The listing builds one solid part. Answer for the finished solid, in the listing's coordinates (mm). A direction names the side the tool comes from. Round coordinates to 2 decimals unless told otherwise and drop trailing zeros. Write each loop counter-clockwise with the first axis right and the second up, starting at its lowest first coordinate (ties: lowest second). Pieces come first, ordered by that corner, then holes.
Item 1: Find section A-A on x = 32. Give the vertices of the cut face in (y, z).
Item 2: Find section C-C on z = 63.5. Give the vertices of the cut face in (x, y).
Item 3: Find section B-B on z = -29.5. Give the vertices of the cut face in (x, y).
Item 4: Each of these flat-tipped pins is pushed along its axis until it touches: pin 1 (5 mm diameter, centred on x = -27, z = 65.5, fed in from -Y); pin 2 (1.1 mm diameter, centred on y = -1.5, z = 48.5, fed in from -X); pin 3 (1.5 mm diameter, centred on x = 4, z = 33.5, fed in from -Y). Where does it stop, or does it pass through?
Item 5: For a pull along X with two mould halves and no side action, classify faces 1 (the face through (-7.703, -1.493, 70.859)), 2 (the face through (-37.64, 5.03, -79.1)), 3 (the face through (0, 9.99, 70)), 4 (the face through (-14, -1, 43)) as +X half, -X half, draft (parallel to the pull), parting line (faces both ways), or undercut.
Item 6: Find the intervals of material crossed by probe 1 along X at (y, z) = (-1.8, 63.5); probe 2 along Y at (x, z) = (31, 72); probe 3 along Y at (x, z) = (-15, 58.5), in increasing order.
Item 7: A tool of negligible diameter and unlimited length cuts with its end or side. For faces 5 (the face through (-31.359, -1.493, 70.797)), 6 (the face through (-19, -2, 51)), 7 (the face through (-25, -1, 64)), from which of +Z, -Z, +X, -X, +Y, -Y can it reach the whole face along a straight path? Write none if from no direction.
```python
from build123d import *

# Parameters (mm, degrees)
SKETCH1_W           = 77
SKETCH1_H           = 160
BOSS_EXTRUDE1_DEPTH = 10
FILLET1_R           = 3
SKETCH2_R           = 2
CUT_EXTRUDE1_DEPTH  = 0.01
BOSS_EXTRUDE2_DEPTH = 2
FILLET2_R           = 1
SKETCH4_R           = 5.25
SKETCH4_R_2         = 3.5
CUT_EXTRUDE2_DEPTH  = 1
SKETCH5_R           = 2
CUT_EXTRUDE3_DEPTH  = 0.01


with BuildPart() as part:
    # Sketch1 → Boss-Extrude1 (new body)
    with BuildSketch(Plane(origin=(0, 0, 0), x_dir=(1, 0, 0), z_dir=(0, 1, 0))):
        Rectangle(SKETCH1_W, SKETCH1_H)
    extrude(amount=BOSS_EXTRUDE1_DEPTH)

    # Fillet1
    fillet1_edges = [part.edges().sort_by_distance(p)[0] for p in [
        (-38.5, 10, 0),
        (0, 10, 80),
        (38.5, 10, 0),
        (0, 0, 80),
        (-38.5, 0, 0),
        (0, 0, -80),
        (38.5, 0, 0),
        (38.5, 5, 80),
        (-38.5, 5, 80),
        (-38.5, 5, -80),
        (38.5, 5, -80),
        (0, 10, -80),
    ]]
    fillet(fillet1_edges, radius=FILLET1_R)

    # Sketch2 → Cut-Extrude1 (cut)
    with BuildSketch(Plane(origin=(0, 10, 0), x_dir=(1, 0, 0), z_dir=(0, 1, 0))):
        with Locations(Location((0, -70, 0), (0, 0, 270))):
            Circle(SKETCH2_R)
    extrude(amount=-CUT_EXTRUDE1_DEPTH, mode=Mode.SUBTRACT)

    # Sketch3 → Boss-Extrude2 (add)
    with BuildSketch(Plane.XZ):
        with BuildLine():
            Line((-28.5, 72), (-10.5, 72))
            ThreePointArc((-10.5, 72), (-7.671572875, 70.828427125), (-6.5, 68))
            Line((-6.5, 68), (-6.5, 34))
            ThreePointArc((-6.5, 34), (-7.671572875, 31.171572875), (-10.5, 30))
            Line((-10.5, 30), (-28.5, 30))
            ThreePointArc((-28.5, 30), (-31.328427125, 31.171572875), (-32.5, 34))
            Line((-32.5, 34), (-32.5, 68))
            ThreePointArc((-32.5, 68), (-31.328427125, 70.828427125), (-28.5, 72))
        make_face()
    extrude(amount=BOSS_EXTRUDE2_DEPTH)

    # Fillet2
    fillet2_edges = [part.edges().sort_by_distance(p)[0] for p in [
        (-31.328427125, 0, 31.171572875),
        (-19.5, 0, 30),
        (-7.671572875, 0, 31.171572875),
        (-6.5, 0, 51),
        (-7.671572875, 0, 70.828427125),
        (-19.5, 0, 72),
        (-31.328427125, 0, 70.828427125),
        (-32.5, 0, 51),
    ]]
    fillet(fillet2_edges, radius=FILLET2_R)

    # Sketch4 → Cut-Extrude2 (cut)
    with BuildSketch(Plane.XZ.offset(2)):
        with Locations(Location((-25.25, 63.5, 0), (0, 0, 270))):
            Circle(SKETCH4_R)
        with Locations(Location((-25.25, 51, 0), (0, 0, 270))):
            Circle(SKETCH4_R)
        with Locations(Location((-25.25, 38.5, 0), (0, 0, 270))):
            Circle(SKETCH4_R)
        with Locations(Location((-12, 57.25, 0), (0, 0, 270))):
            Circle(SKETCH4_R_2)
        with Locations(Location((-12, 44.75, 0), (0, 0, 270))):
            Circle(SKETCH4_R_2)
    extrude(amount=-CUT_EXTRUDE2_DEPTH, mode=Mode.SUBTRACT)

    # Sketch5 → Cut-Extrude3 (cut)
    with BuildSketch(Plane.XZ.offset(1)):
        with Locations(Location((-12, 44.75, 0), (0, 0, 270))):
            Circle(SKETCH5_R)
    extrude(amount=-CUT_EXTRUDE3_DEPTH, mode=Mode.SUBTRACT)


solid = part.part
```
Check values:
1. outline: (0, -77) arc R3 ccw to (3, -80) - (7, -80) arc R3 ccw to (10, -77) - (10, 77) arc R3 ccw to (7, 80) - (3, 80) arc R3 ccw to (0, 77) - close
2. outline: (-38.5, 3) arc R3 ccw to (-35.5, 0) - (-33.5, 0) arc R1 cw to (-32.5, -1) - (-32.5, -2) - (-30.5, -2) - (-30.5, -1) - (-20, -1) - (-20, -2) - (-6.5, -2) - (-6.5, -1) arc R1 cw to (-5.5, 0) - (35.5, 0) arc R3 ccw to (38.5, 3) - (38.5, 7) arc R3 ccw to (35.5, 10) - (-35.5, 10) arc R3 ccw to (-38.5, 7) - close
3. outline: (-38.5, 3) arc R3 ccw to (-35.5, 0) - (35.5, 0) arc R3 ccw to (38.5, 3) - (38.5, 7) arc R3 ccw to (35.5, 10) - (-35.5, 10) arc R3 ccw to (-38.5, 7) - close
4. pin 1: stops at y = -1
4. pin 2: stops at x = -32.5
4. pin 3: stops at y = 0
5. face 1: +X half
5. face 2: -X half
5. face 3: draft
5. face 4: undercut
6. probe 1: x = -32.5 to -30.5, -20 to -6.5
6. probe 2: y = 0 to 10
6. probe 3: y = -1 to 10
7. face 5: +Z, -X, -Y
7. face 6: +Z, -Z, +X, -X, -Y
7. face 7: -Y
